```python
from build123d import *

# Parameters (mm, degrees)
F1_DEPTH = 10
F2_R     = 1.6
F3_DEPTH = 25
F2_R_2   = 3
F4_DEPTH = 2.3
F5_R     = 3


with BuildPart() as f1:
    # F0 (on Front) → F1 (new body)
    with BuildSketch(Plane.XZ):
        Polygon((12, -3.5), (14, -3.5), (14, 3.5), (-14, 3.5), (-14, -3.5), (-12, -3.5), (-12, -2), (-10, -2), (-10, -3.5), (-8, -3.5), (-8, -2), (-6, -2), (-6, -3.5), (-4, -3.5), (-4, -2), (-2, -2), (-2, -3.5), (2, -3.5), (2, -2), (4, -2), (4, -3.5), (6, -3.5), (6, -2), (8, -2), (8, -3.5), (10, -3.5), (10, -2), (12, -2), align=None)
    extrude(amount=F1_DEPTH)

    # F2 (on face) → F3 (cut)
    with BuildSketch(Plane.XY.offset(3.5)):
        with Locations((0, -5)):
            Circle(F2_R)
    extrude(amount=-F3_DEPTH, mode=Mode.SUBTRACT)

    # F2 (on face) → F4 (cut)
    with BuildSketch(Plane.XY.offset(3.5)):
        with Locations((0, -5)):
            Circle(F2_R_2)
        with Locations((0, -5)):
            Circle(F2_R, mode=Mode.SUBTRACT)
    extrude(amount=-F4_DEPTH, mode=Mode.SUBTRACT)

    # F5
    f5_edges = [f1.edges().sort_by_distance(p)[0] for p in [
        (-14, -5, 3.5),
        (14, -5, 3.5),
    ]]
    fillet(f5_edges, radius=F5_R)


solid = f1.part
```
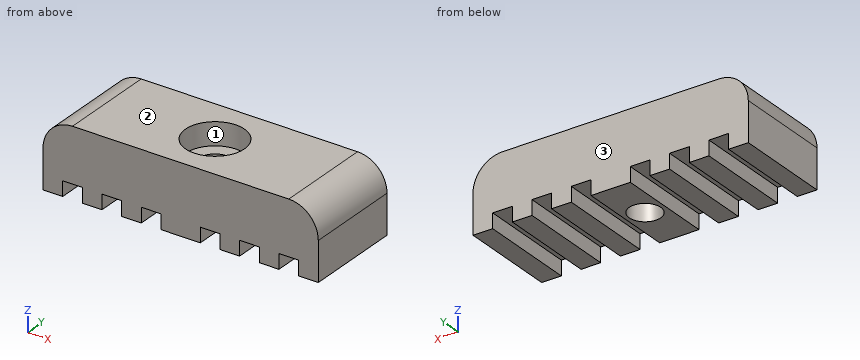
Read the model definition and answer for the solid it produces. Units are mm, in the model's axes. Face numbers are marked on the shaded views. Coordinates: 2 decimals unless noted, no trailing zeros. Loops run counter-clockwise (first coordinate to the right, second up) from the corner with the lowest first, then second, coordinate; pieces in that order, holes last.
(1) Flat-ended cylindrical pins translate along their axes: pin 1 Ø3.5 at (x, y) = (0, -5) entering from +Z; pin 2 Ø3 at (x, y) = (0, -5) entering from +Z. Find the tip coordinate at first contact, or state that the pin passes through.
Solution:
pin 1: stops at z = 1.2
pin 2: passes through
(2) The part is cut by section C-C (z = 0.25). Determine the outline of the cut face in (x, y), and give its area (3 significant figures).
Solution:
outline: (-14, -10) - (14, -10) - (14, 0) - (-14, 0) - close; hole circle Ø3.2 at (0, -5)
area: 272 mm2
(3) The part is cut by section B-B (z = -2.5). Count the separate pieces of the cut face and the enclosed holes in it, and give its area (3 significant figures).
Solution:
separate pieces: 7
enclosed holes: 1
area: 152 mm2
(4) The part is cut by section A-A (x = 0). Determine the outline of the cut face in (y, z), and give its area (3 significant figures).
Solution:
outline: (-10, -3.5) - (-6.6, -3.5) - (-6.6, 1.2) - (-8, 1.2) - (-8, 3.5) - (-10, 3.5) - close; (-3.4, -3.5) - (0, -3.5) - (0, 3.5) - (-2, 3.5) - (-2, 1.2) - (-3.4, 1.2) - close
area: 41.2 mm2
(5) Consider line 1 along Y through (x, z) = (0, 1.25); line 2 along Z through (x, y) = (-6.75, -6.25); line 3 along Y through (x, z) = (0, -0.1). Determine where each line is inside the solid, lowest interval first.
Solution:
line 1: y = -10 to -8, -2 to 0
line 2: z = -2 to 3.5
line 3: y = -10 to -6.6, -3.4 to 0
(6) The mould has two halves that part along Y. Classify the marked faces 1, 2 and 3: released by +Y, released by -Y, zero draft, split by the parting line, or undercut.
Solution:
face 1: undercut
face 2: zero draft
face 3: released by +Y
